Here's the drawing with two shaded views (mm, measured from the low corner). I have some questions. A direction names the side the tool comes from. Round coordinates to 2 decimals unless told otherwise and drop trailing zeros. Order: outer loops, then holes, each group sorted by start corner. A loop starts at its lowest first (then second) coordinate and runs counter-clockwise, first axis right, second up. Notation, with made-up numbers: (51.5, -22) -> (56.5, -22) arc R8 cw to (56.5, -17) -> close; hole circle Ø8 at (4, 33). An arc over 180 degrees is marked (long way). Use a Markdown table: item, result. Add a question column.
Q1. For the marked faces 1 and 2, which set-ups out of +Z, -Z, +X, -X, +Y, -Y let a thin tool reach every point of the face, with its end or its side?
Q2. I need wall thicknesses on line 1 along X through (y, z) = (29, 49); line 2 along Y through (x, z) = (12.7, 49.75) (3 decimals); line 3 along Y through (x, z) = (4.25, 22). Which ranges of each line are inside material? Lowest first, please. Write a range as [from, to].
Q3. If we section it at A-A on x = 12.7: List the corners of the cut face in (y, z) for me (3 decimals).
Q4. If we section it at C-C on z = 21.59: List the corners of the cut face in (x, y) for me (3 decimals), plus the area to 3 significant figures.
Q5. If we section it at D-D on x = 18.5: List the corners of the cut face in (y, z) for me (3 decimals), plus the area to 3 significant figures.
Q6. I'm going to push flat-ended pins straight in: pin 1 Ø6 at (x, y) = (2.5, 25.5) entering from -Z; pin 2 Ø6 at (x, z) = (5, 43) entering from +Y. Where does each tip first touch, or does it pass through?
Q7. If we section it at B-B on y = 29.21: List the corners of the cut face in (x, z) for me (3 decimals), plus the area to 3 significant figures.
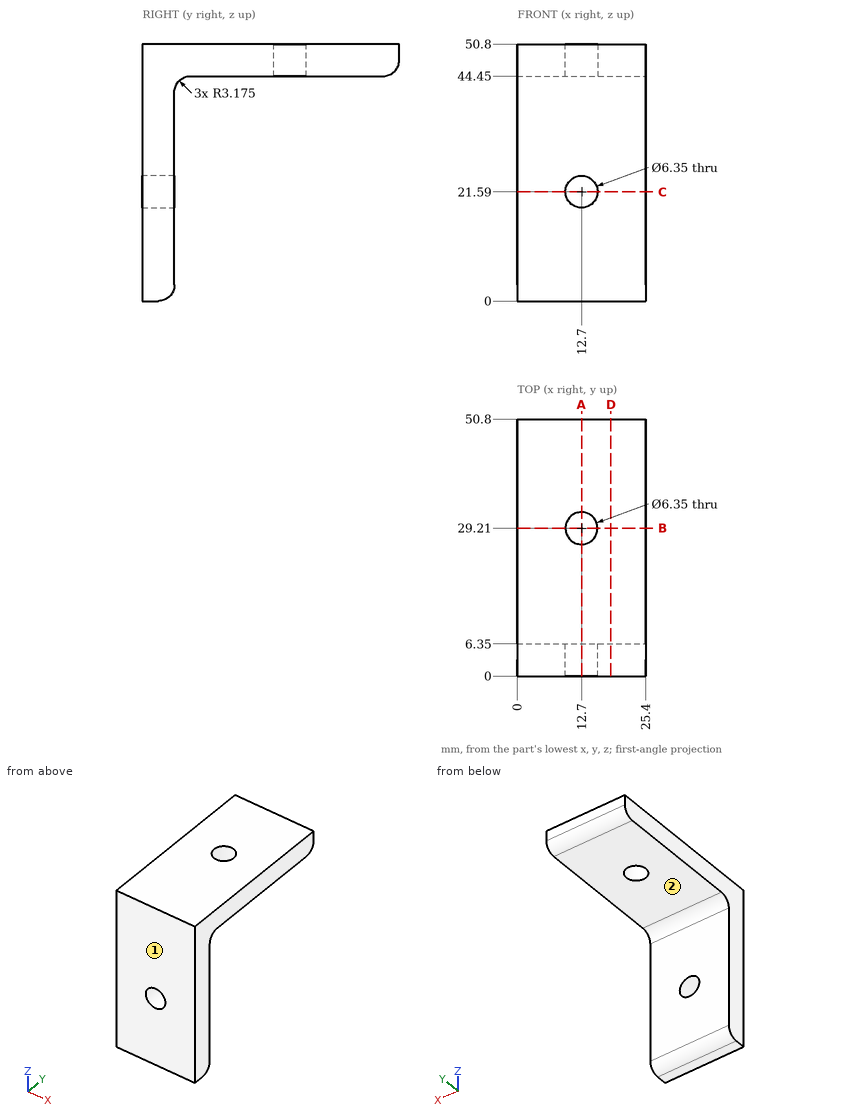
Answer below:
| question | item | result |
|---|---|---|
| 1 | face 1 | +Z, -Z, +X, -X, -Y |
| 1 | face 2 | -Z, +X, -X, +Y |
| 2 | line 1 | [0, 9.53], [15.87, 25.4] |
| 2 | line 2 | [0, 26.035], [32.385, 50.8] |
| 2 | line 3 | [0, 6.35] |
| 3 | outline | (0, 0) -> (3.175, 0) arc R3.175 ccw to (6.35, 3.175) -> (6.35, 18.415) -> (0, 18.415) -> close; (0, 24.765) -> (6.35, 24.765) -> (6.35, 41.275) arc R3.175 cw to (9.525, 44.45) -> (26.035, 44.45) -> (26.035, 50.8) -> (0, 50.8) -> close; (32.385, 44.45) -> (47.625, 44.45) arc R3.175 ccw to (50.8, 47.625) -> (50.8, 50.8) -> (32.385, 50.8) -> close |
| 4 | outline | (0, 0) -> (9.525, 0) -> (9.525, 6.35) -> (0, 6.35) -> close; (15.875, 0) -> (25.4, 0) -> (25.4, 6.35) -> (15.875, 6.35) -> close |
| 4 | area | 121 mm² |
| 5 | outline | (0, 0) -> (3.175, 0) arc R3.175 ccw to (6.35, 3.175) -> (6.35, 41.275) arc R3.175 cw to (9.525, 44.45) -> (47.625, 44.45) arc R3.175 ccw to (50.8, 47.625) -> (50.8, 50.8) -> (0, 50.8) -> close |
| 5 | area | 603 mm² |
| 6 | pin 1 | z = 44.45 |
| 6 | pin 2 | y = 50.35 |
| 7 | outline | (0, 44.45) -> (9.525, 44.45) -> (9.525, 50.8) -> (0, 50.8) -> close; (15.875, 44.45) -> (25.4, 44.45) -> (25.4, 50.8) -> (15.875, 50.8) -> close |
| 7 | area | 121 mm² |
